Here's the drawing with two shaded views (mm, measured from the low corner). I have some questions. A direction names the side the tool comes from. Round coordinates to 2 decimals unless told otherwise and drop trailing zeros. Order: outer loops, then holes, each group sorted by start corner. A loop starts at its lowest first (then second) coordinate and runs counter-clockwise, first axis right, second up.
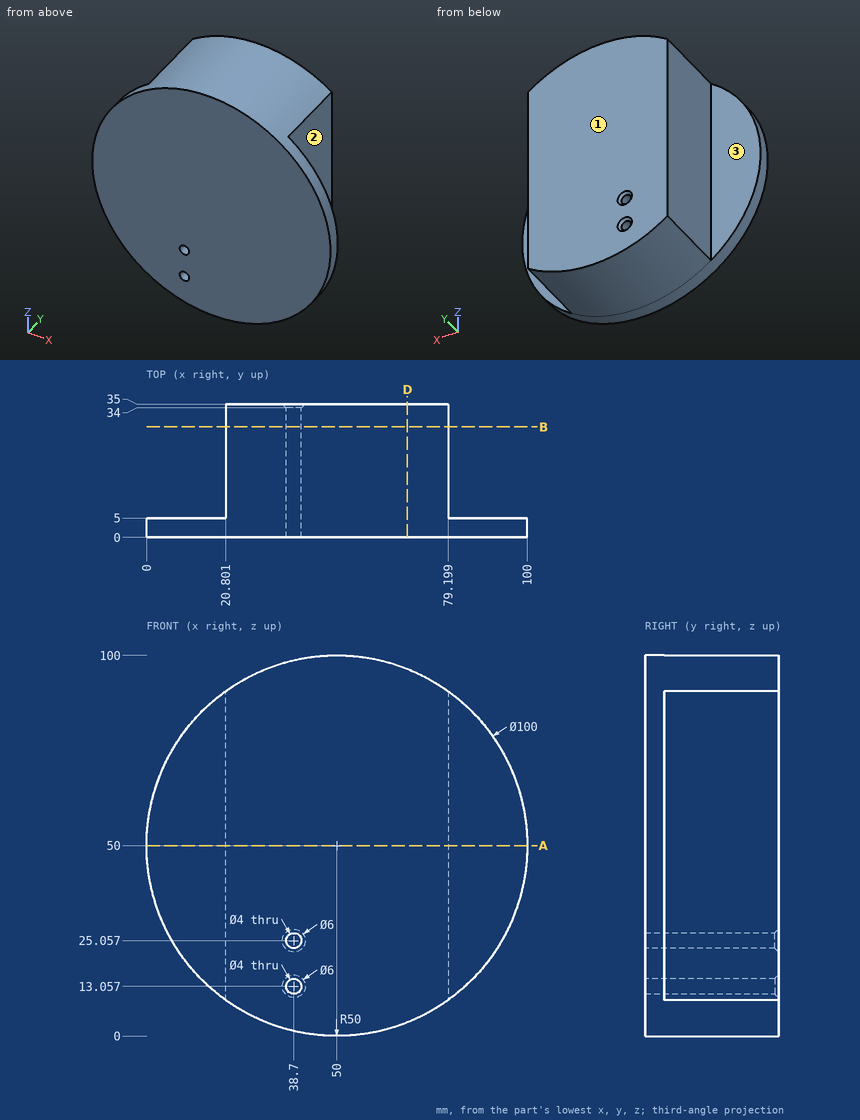
1. If we section it at A-A, the plane z = 50: Write out the boundary of the cut face in (x, y), and give its area (3 significant figures).
Evaluation:
outline: (0, 0) - (100, 0) - (100, 5) - (79.2, 5) - (79.2, 35) - (20.8, 35) - (20.8, 5) - (0, 5) - close
area: 2,250 mm2
2. I need wall thicknesses on probe 1 along Z at (x, y) = (38, 16); probe 2 along Y at (x, z) = (41.5, 12); probe 3 along Y at (x, z) = (20, 25.5). Which ranges of each line are inside material? Lowest first, please.
Evaluation:
probe 1: z = 1.46 to 11.18, 14.93 to 23.18, 26.93 to 98.54
probe 2: y = 0 to 34.99
probe 3: y = 0 to 5
3. On a 3-axis mill with a long thin cutter (end or side, diameter ignored), from which of +Z, -Z, +X, -X, +Y, -Y can I reach the whole of each face in a straight line? I mean the marked faces 1, 2 and 3. Say none if no direction works.
Evaluation:
face 1: +Z, -Z, +X, -X, +Y
face 2: +Z, -Z, +X, +Y
face 3: +Z, -Z, -X, +Y
4. I'm going to push flat-ended pins straight in: P1, Ø12, axis at y = 16.5, z = 25, coming from the -X side; P2, Ø9, axis at y = 13.5, z = 38, coming from the +X side; P3, Ø23, axis at x = 93, z = 66.5, coming from the +Y side; P4, Ø4.5, axis at x = 38.7, z = 13.06, coming from the -Y side. Where does each tip first touch, or does it pass through?
Evaluation:
P1: stops at x = 20.8
P2: stops at x = 79.2
P3: stops at y = 5
P4: stops at y = 0
5. If we section it at D-D, the plane x = 68.5: Write out the boundary of the cut face in (y, z).
Evaluation:
outline: (0, 3.55) - (35, 3.55) - (35, 96.45) - (0, 96.45) - close
6. If we section it at B-B, the plane y = 29: Write out the boundary of the cut face in (x, z), and give its area (3 significant figures).
Evaluation:
outline: (20.8, 9.41) arc R50 ccw to (79.2, 9.41) - (79.2, 90.59) arc R50 ccw to (20.8, 90.59) - close; hole circle Ø4 at (38.7, 13.06); hole circle Ø4 at (38.7, 25.06)
area: 5,460 mm2
